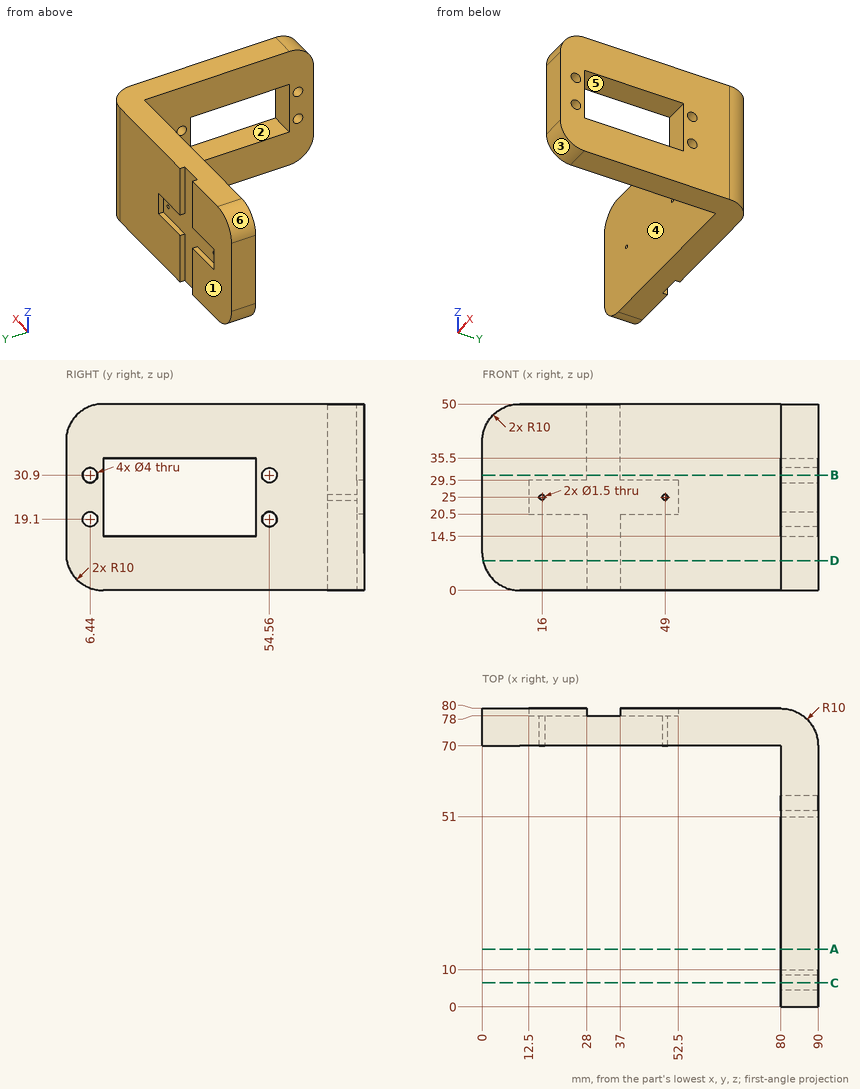
Answer from the drawing. Dimensions are ordinates in mm from the lowest x, y and z of the part. A direction names the side the tool comes from. Give positions to 0.01 mm unless a question says otherwise; leave off trailing zeros. Order: outer loops, then holes, each group sorted by start corner. A loop starts at its lowest first (then second) coordinate and runs counter-clockwise, first axis right, second up. Notation, with made-up numbers: (61.5, -33.75) -> (114.5, -33.75) arc R23 ccw to (114.5, -22.75) -> close; hole circle Ø5 at (-16, -37). An arc over 180 degrees is marked (long way). One line per item, written item: value.
Item 1: Determine the mould class of the marked faces 1, 2 and 3 for opening direction Z: released by +Z, released by -Z, zero draft, split by the parting line, or undercut.
Answer sheet:
face 1: zero draft
face 2: undercut
face 3: released by -Z
Item 2: Straight lines are drawn through the part: probe 1 along Z at (x, y) = (84.5, 54.56); probe 2 along X at (y, z) = (74.5, 25); probe 3 along Z at (x, y) = (49, 71). For each, find the intervals that lie inside material, in ascending order.
Answer sheet:
probe 1: 0 to 17.1, 21.1 to 28.9, 32.9 to 50
probe 2: 0 to 15.25, 16.75 to 48.25, 49.75 to 88.93
probe 3: 0 to 24.25, 25.75 to 50
Item 3: Flat-ended cylindrical pins translate along their axes: P1, Ø2, axis at x = 70.5, z = 31.5, coming from the -Y side; P2, Ø2, axis at y = 79, z = 11.5, coming from the +X side; P3, Ø2, axis at x = 16, z = 25, coming from the +Y side. Find the tip coordinate at first contact, or state that the pin passes through.
Answer sheet:
P1: y = 70
P2: x = 86
P3: y = 78
Item 4: Find section B-B, the plane z = 30.9. Give the vertices of the cut face in (x, y), plus the area to 3 significant figures.
Answer sheet:
outline: (0, 70) -> (80, 70) -> (80, 56.56) -> (90, 56.56) -> (90, 70) arc R10 ccw to (80, 80) -> (37, 80) -> (37, 78) -> (28, 78) -> (28, 80) -> (0, 80) -> close; (80, 0) -> (90, 0) -> (90, 4.44) -> (80, 4.44) -> close; (80, 8.44) -> (90, 8.44) -> (90, 10) -> (80, 10) -> close; (80, 51) -> (90, 51) -> (90, 52.56) -> (80, 52.56) -> close
area: 1,070 mm²
Item 5: Find section D-D, the plane z = 8. Give the vertices of the cut face in (x, y), plus the area to 3 significant figures.
Answer sheet:
outline: (0.2, 70) -> (80, 70) -> (80, 0.2) -> (90, 0.2) -> (90, 70) arc R10 ccw to (80, 80) -> (37, 80) -> (37, 78) -> (28, 78) -> (28, 80) -> (0.2, 80) -> close
area: 1,560 mm²
Item 6: Find section C-C, the plane y = 6.44. Give the vertices of the cut face in (x, z), plus the area to 3 significant figures.
Answer sheet:
outline: (80, 0.66) -> (90, 0.66) -> (90, 17.1) -> (80, 17.1) -> close; (80, 21.1) -> (90, 21.1) -> (90, 28.9) -> (80, 28.9) -> close; (80, 32.9) -> (90, 32.9) -> (90, 49.34) -> (80, 49.34) -> close
area: 407 mm²
Item 7: Find section A-A, the plane y = 15.5. Give the vertices of the cut face in (x, z), plus the area to 3 significant figures.
Answer sheet:
outline: (80, 0) -> (90, 0) -> (90, 14.5) -> (80, 14.5) -> close; (80, 35.5) -> (90, 35.5) -> (90, 50) -> (80, 50) -> close
area: 290 mm²
Item 8: A tool of negligible diameter and unlimited length cuts with its end or side. For the marked faces 4, 5 and 6, from which of +Z, -Z, +X, -X, +Y, -Y can it reach the whole face along a straight path? Write none if from no direction.
Answer sheet:
face 4: +Z, -Z, -X, -Y
face 5: +X, -X
face 6: +Z, -X, +Y, -Y
